from build123d import *

# Parameters (mm, degrees)
BOSS_EXTRUDE1_DEPTH = 3
BOSS_EXTRUDE2_DEPTH = 3
SKETCH3_W           = 17
SKETCH3_H           = 13
SKETCH3_R           = 2.15
SKETCH3_R_2         = 0.75
BOSS_EXTRUDE3_DEPTH = 3
CUT_EXTRUDE2_REACH  = 32.336
SKETCH6_R           = 2.15
CUT_EXTRUDE3_REACH  = 33.02
SKETCH8_R           = 1.75
SKETCH4_R           = 1.75
CUT_EXTRUDE4_DEPTH  = 1.2


with BuildPart() as part:
    # Sketch1 → Boss-Extrude1 (new body)
    with BuildSketch(Plane.XY):
        Polygon((0, 0), (17, 0), (21.5, 0), (21.5, 4.5), (17, 4.5), (17, 20), (0, 20), (-4.5, 20), (-4.5, 15.5), (0, 15.5), align=None)
    extrude(amount=BOSS_EXTRUDE1_DEPTH)

    # Sketch2 → Boss-Extrude2 (add)
    with BuildSketch(Plane.XY.offset(3)):
        Polygon((0, 20), (0, 15.5), (0, 0), (2, 0), (2, 17), (15, 17), (15, 0), (17, 0), (17, 20), align=None)
    extrude(amount=BOSS_EXTRUDE2_DEPTH)

    # Sketch3 → Boss-Extrude3 (add)
    with BuildSketch(Plane(origin=(0, 20, 0), x_dir=(1, 0, 0), z_dir=(0, 1, 0))):
        with Locations((8.5, -6.5)):
            Rectangle(SKETCH3_W, SKETCH3_H)
        with Locations((8.5, -8)):
            Circle(SKETCH3_R, mode=Mode.SUBTRACT)
        with Locations(Location((13, -8, 0), (0, 0, 270))):
            Circle(SKETCH3_R_2, mode=Mode.SUBTRACT)
        with Locations(Location((4, -8, 0), (0, 0, 270))):
            Circle(SKETCH3_R_2, mode=Mode.SUBTRACT)
    extrude(amount=-BOSS_EXTRUDE3_DEPTH)

    # Sketch6 → Cut-Extrude2 (cut, up to next)
    with BuildSketch(Plane(origin=(0, 17, 0), x_dir=(-1, 0, 0), z_dir=(0, -1, 0)), mode=Mode.PRIVATE) as cut_extrude2_sk1:
        with Locations(Location((-8.5, -8, 0), (0, 0, 270))):
            Circle(SKETCH6_R)
    cut_extrude2_tool1 = extrude(cut_extrude2_sk1.sketch, amount=-CUT_EXTRUDE2_REACH, mode=Mode.PRIVATE) & part.part
    add(cut_extrude2_tool1.solids().sort_by_distance((8.5, 17, 8))[0], mode=Mode.SUBTRACT)

    # Sketch8 → Cut-Extrude3 (cut, up to next)
    with BuildSketch(Plane.XY.offset(3), mode=Mode.PRIVATE) as cut_extrude3_sk1:
        with Locations((19.25, 2.25)):
            Circle(SKETCH8_R)
    cut_extrude3_tool1 = extrude(cut_extrude3_sk1.sketch, amount=-CUT_EXTRUDE3_REACH, mode=Mode.PRIVATE) & part.part
    # Sketch8 → Cut-Extrude3 (cut, up to next)
    with BuildSketch(Plane.XY.offset(3), mode=Mode.PRIVATE) as cut_extrude3_sk2:
        with Locations((-2.25, 17.75)):
            Circle(SKETCH8_R)
    cut_extrude3_tool2 = extrude(cut_extrude3_sk2.sketch, amount=-CUT_EXTRUDE3_REACH, mode=Mode.PRIVATE) & part.part
    add(cut_extrude3_tool1.solids().sort_by_distance((19.25, 2.25, 3))[0], mode=Mode.SUBTRACT)
    add(cut_extrude3_tool2.solids().sort_by_distance((-2.25, 17.75, 3))[0], mode=Mode.SUBTRACT)

    # Sketch4 → Cut-Extrude4 (cut)
    with BuildSketch(Plane(origin=(0, 20, 0), x_dir=(-1, 0, 0), z_dir=(0, -1, 0))):
        with Locations(Location((-4, -8, 0), (0, 0, 90))):
            Circle(SKETCH4_R)
        with Locations(Location((-13, -8, 0), (0, 0, 90))):
            Circle(SKETCH4_R)
    extrude(amount=CUT_EXTRUDE4_DEPTH, mode=Mode.SUBTRACT)


solid = part.part
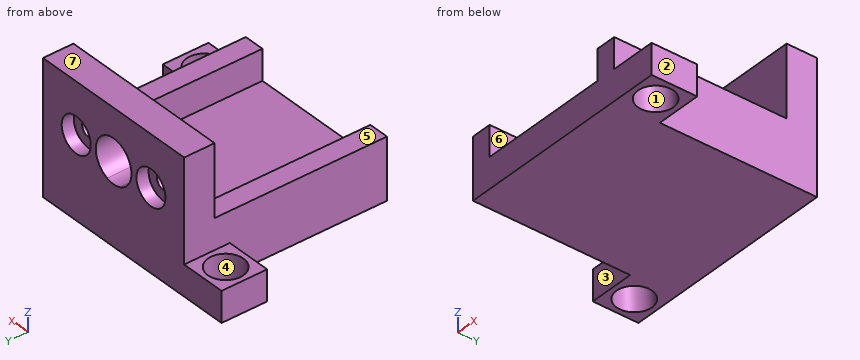
Geometry: final body of the model. Coordinates: model frame, mm. Face numbers are marked on the shaded views. A direction names the side the tool comes from. Round coordinates to 2 decimals unless told otherwise and drop trailing zeros. Loops run counter-clockwise (first coordinate to the right, second up) from the corner with the lowest first, then second, coordinate; pieces in that order, holes last. Notation, with made-up numbers: (-40, 42.5) -> (8, 42.5) arc R7 ccw to (8, 51.5) -> close; hole circle Ø5 at (-11.75, -8.75). An arc over 180 degrees is marked (long way). One line per question, with ' | ' between items. Start each with the question number.
1. Section C-C on y = 2.75. Output: boundary loops of the cut face in (x, z).
2. Section D-D on x = -2.25. Output: boundary loops of the cut face in (y, z), and give its area (3 significant figures).
3. Contact query for flat-ended pins moving along their axis: pin 1 (2 mm diameter, centred on x = 16, y = 8.5, fed in from +Z); pin 2 (2.5 mm diameter, centred on y = 9, z = 4, fed in from +X); pin 3 (4 mm diameter, centred on x = 8, y = 2.5, fed in from +Z); pin 4 (1.4 mm diameter, centred on x = 4, z = 8, fed in from +Y). Output: stop coordinate, or through.
4. Line query: line 1 along X through (y, z) = (19.5, 8); line 2 along Y through (x, z) = (19.25, 0.95); line 3 along X through (y, z) = (4.25, 5.25). Output: solid intervals per line, ascending. Write a range as [from, to].
5. Mould query, pull axis Y, two halves, no side actions, for the marked faces 1, 2, 3 and 4. Classes: pulls with the +Y half, pulls with the -Y half, needs draft (parallel to the pull), parting line crosses it, or undercut.
6. Set-up query: the marked faces 5, 6 and 7. Return all of +Z, -Z, +X, -X, +Y, -Y with unobstructed straight access to the full face (end or side cutting, diameter ignored); none if empty.
7. Section B-B on z = 8. Output: boundary loops of the cut face in (x, y).
8. Section A-A on x = 4. Output: boundary loops of the cut face in (y, z), and give its area (3 significant figures).
Returned:
1) outline: (0, 0) -> (17.57, 0) -> (17.57, 3) -> (17, 3) -> (17, 6) -> (15, 6) -> (15, 3) -> (2, 3) -> (2, 6) -> (0, 6) -> close; (20.93, 0) -> (21.5, 0) -> (21.5, 3) -> (20.93, 3) -> close
2) outline: (15.5, 0) -> (16, 0) -> (16, 3) -> (15.5, 3) -> close; (19.5, 0) -> (20, 0) -> (20, 3) -> (19.5, 3) -> close | area: 3.00 mm2
3) pin 1: stops at z = 6 | pin 2: stops at x = 17 | pin 3: stops at z = 3 | pin 4: passes through
4) line 1: x = [0, 2.25], [5.75, 6.35], [10.65, 11.25], [14.75, 17] | line 2: y = [0, 0.5], [4, 4.5] | line 3: x = [0, 2], [15, 17]
5) face 1: undercut | face 2: needs draft | face 3: pulls with the -Y half | face 4: undercut
6) face 5: +Z, +X, -X, -Y | face 6: +Z, -Y | face 7: +Z, +X, -X, +Y, -Y
7) outline: (0, 17) -> (3.25, 17) -> (3.25, 18.8) -> (2.25, 18.8) -> (2.25, 20) -> (0, 20) -> close; (4.75, 17) -> (6.35, 17) -> (6.35, 20) -> (5.75, 20) -> (5.75, 18.8) -> (4.75, 18.8) -> close; (10.65, 17) -> (12.25, 17) -> (12.25, 18.8) -> (11.25, 18.8) -> (11.25, 20) -> (10.65, 20) -> close; (13.75, 17) -> (17, 17) -> (17, 20) -> (14.75, 20) -> (14.75, 18.8) -> (13.75, 18.8) -> close
8) outline: (0, 0) -> (20, 0) -> (20, 6.25) -> (18.8, 6.25) -> (18.8, 7.25) -> (17, 7.25) -> (17, 3) -> (0, 3) -> close; (17, 8.75) -> (18.8, 8.75) -> (18.8, 9.75) -> (20, 9.75) -> (20, 13) -> (17, 13) -> close | area: 83.1 mm2
